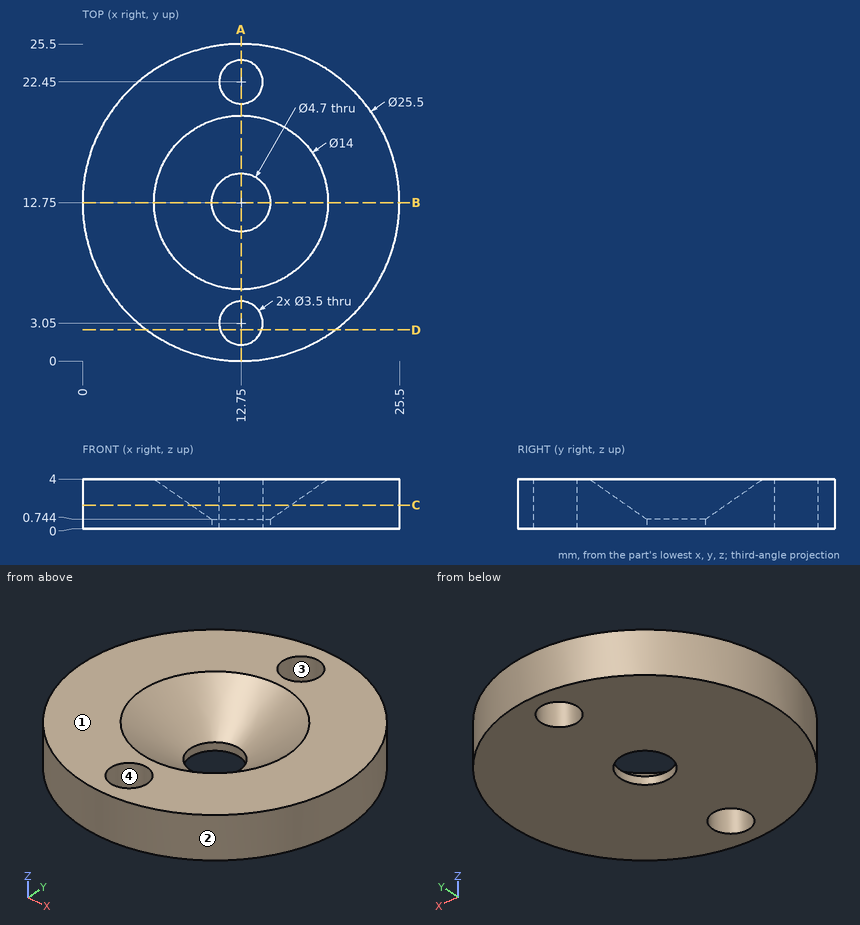
Answer from the drawing. Dimensions are ordinates in mm from the lowest x, y and z of the part. Give positions to 0.01 mm unless a question says otherwise; leave off trailing zeros. Loops run counter-clockwise (first coordinate to the right, second up) from the corner with the lowest first, then second, coordinate; pieces in that order, holes last. Notation, with made-up numbers: (64.5, 66) -> (88.5, 66) arc R32 cw to (88.5, 98) -> close; hole circle Ø10 at (67, 72). An arc over 180 degrees is marked (long way). One line per question, with ' | ' between items. Start each with the question number.
1) Section B-B, the plane y = 12.75 is taken. Determine the outline of the cut face in (x, z).
2) Section A-A, the plane x = 12.75 is taken. Determine the outline of the cut face in (y, z).
3) Determine the mould class of the marked faces 1, 2, 3 and 4 for opening direction Y: +Y half, -Y half, draft (parallel to the pull), parting line (faces both ways), or undercut.
4) Section C-C, the plane z = 1.9 is taken. Determine the outline of the cut face in (x, y), then the cut area to 3 significant figures.
5) Section D-D, the plane y = 2.5 is taken. Determine the outline of the cut face in (x, z), then the cut area to 3 significant figures.
6) Straight lines are drawn through the part: L1, parallel to Y at x = 12.75, z = 0.65; L2, parallel to Y at x = 12.75, z = 1.7 (1 decimal); L3, parallel to X at y = 13, z = 1.7. For each, find the intervals that lie inside material, in ascending order.
7) Each of these flat-tipped pins is pushed along its axis until it touches: pin 1 (8 mm diameter, centred on x = 15, y = 12, fed in from +Z); pin 2 (3 mm diameter, centred on x = 12.75, y = 3.05, fed in from -Z); pin 3 (2 mm diameter, centred on x = 22, z = 1.5, fed in from +Y). Where does it stop, or does it pass through?
Resolved:
1) outline: (0, 0) -> (10.4, 0) -> (10.4, 0.74) -> (5.75, 4) -> (0, 4) -> close; (15.1, 0) -> (25.5, 0) -> (25.5, 4) -> (19.75, 4) -> (15.1, 0.74) -> close
2) outline: (0, 0) -> (1.3, 0) -> (1.3, 4) -> (0, 4) -> close; (4.8, 0) -> (10.4, 0) -> (10.4, 0.74) -> (5.75, 4) -> (4.8, 4) -> close; (15.1, 0) -> (20.7, 0) -> (20.7, 4) -> (19.75, 4) -> (15.1, 0.74) -> close; (24.2, 0) -> (25.5, 0) -> (25.5, 4) -> (24.2, 4) -> close
3) face 1: draft | face 2: parting line | face 3: undercut | face 4: undercut
4) outline: circle Ø25.5 at (12.75, 12.75); hole circle Ø8 at (12.75, 12.75); hole circle Ø3.5 at (12.75, 3.05); hole circle Ø3.5 at (12.75, 22.45) | area: 441 mm2
5) outline: (5.17, 0) -> (11.09, 0) -> (11.09, 4) -> (5.17, 4) -> close; (14.41, 0) -> (20.33, 0) -> (20.33, 4) -> (14.41, 4) -> close | area: 47.4 mm2
6) L1: 0 to 1.3, 4.8 to 10.4, 15.1 to 20.7, 24.2 to 25.5 | L2: 0 to 1.3, 4.8 to 9, 16.5 to 20.7, 24.2 to 25.5 | L3: 0 to 9.04, 16.46 to 25.5
7) pin 1: z = 3.56 | pin 2: through | pin 3: y = 22.47
